Source: CAD feature listing. Evaluate the final solid. Frame: model axes, mm. Face numbers are marked on the shaded views. A direction names the side the tool comes from. Round coordinates to 2 decimals unless told otherwise and drop trailing zeros. Order: outer loops, then holes, each group sorted by start corner. A loop starts at its lowest first (then second) coordinate and runs counter-clockwise, first axis right, second up. Notation, with made-up numbers: M 30.5,89.25 L 59.5,89.25 A23 cw 59.5,126.25 Z; hole C 68,32.5 d9. An arc over 180 degrees is marked long. Answer as CSV lines item,"result". Start each with the question number.
Item 1: Section query B-B on z = 2.5. Return the cut outline in (x, y).
Item 2: Section query C-C on x = -8. Return the cut outline in (y, z), plus the area to 3 significant figures.
Item 3: Line query: line 1 (Y direction, x = 0, z = 37.5); line 2 (X direction, y = 4, z = 0); line 3 (X direction, y = 72, z = 22). Output: solid intervals per line, ascending. Write a range as [from, to].
Item 4: Section query A-A on x = -2.5. Return the cut outline in (y, z), plus the area to 3 significant figures.
Item 5: Section query D-D on y = 52.5. Return the cut outline in (x, z).
Item 6: Set-up query: the marked faces 1 and 2. Return all of +Z, -Z, +X, -X, +Y, -Y with unobstructed straight access to the full face (end or side cutting, diameter ignored); none if empty.
Item 7: First-contact query: P1, Ø10, axis at x = -1, y = 72.5, coming from the +Z side; P2, Ø8, axis at y = 36.5, z = -8.5, coming from the +X side; P3, Ø1, axis at x = -7.5, y = 29, coming from the +Z side. Flat tips, straight axial feed; report the tip coordinate or a pass-through.
Item 8: Pull-direction query (X, two-part tool) for the marked faces 3, 4 and 5; classes: +X half, -X half, draft (parallel to the pull), parting line (faces both ways), or undercut.
from build123d import *
from build123d.topology import SkipClean

# Parameters (mm, degrees)
SKETCH1_R           = 15.3
BOSS_EXTRUDE1_DEPTH = 84.864
SKETCH2_R           = 13.97
BOSS_EXTRUDE2_DEPTH = 57.15
BOSS_EXTRUDE3_DEPTH = 2.54
SKETCH4_R           = 10.2235
CUT_EXTRUDE1_DEPTH  = 5.08
SKETCH5_R           = 14.2621
SKETCH5_R_2         = 10.2235
BOSS_EXTRUDE4_DEPTH = 19.05
SKETCH6_R           = 10.75
CUT_EXTRUDE2_DEPTH  = 6.2
SKETCH8_R           = 14.2621
CUT_EXTRUDE5_DEPTH  = 10.16
SKETCH10_R          = 13.97
BOSS_EXTRUDE5_DEPTH = 24.13
SKETCH11_R          = 10.2235
CUT_EXTRUDE7_DEPTH  = 41.91
SKETCH13_R          = 14.2621
SKETCH13_R_2        = 10.2235
CUT_EXTRUDE9_DEPTH  = 41.91
SKETCH16_R          = 13.97
SKETCH16_R_2        = 10.2235
CUT_EXTRUDE10_DEPTH = 27.78125
SKETCH17_R          = 10.2235
CUT_EXTRUDE11_DEPTH = 27.686
SKETCH18_R          = 6.35
CUT_EXTRUDE12_DEPTH = 111.506


with BuildPart() as part:
    # Sketch1 → Boss-Extrude1 (new body)
    with BuildSketch(Plane(origin=(0, 0, 0), x_dir=(1, 0, 0), z_dir=(0, 1, 0))):
        with Locations(Location((0, 0, 0), (0, 0, 270))):
            Circle(SKETCH1_R)
    extrude(amount=BOSS_EXTRUDE1_DEPTH)

    # Sketch2 → Boss-Extrude2 (add)
    with BuildSketch(Plane.XY):
        with Locations(Location((0, 70.894, 0), (0, 0, 269.999999993))):
            Circle(SKETCH2_R)
    extrude(amount=BOSS_EXTRUDE2_DEPTH)

    # Sketch3 → Boss-Extrude3 (add, symmetric)
    with BuildSketch(Plane.XY.offset(57.15)):
        with BuildLine():
            Line((16.764, 70.894), (16.764, 40.838899717))
            ThreePointArc((16.764, 40.838899717), (0, 24.074899717), (-16.764, 40.838899717))
            Line((-16.764, 40.838899717), (-16.764, 70.894))
            ThreePointArc((-16.764, 70.894), (0, 87.658), (16.764, 70.894))
        make_face()
    extrude(amount=BOSS_EXTRUDE3_DEPTH, both=True)

    # Sketch4 → Cut-Extrude1 (cut)
    with BuildSketch(Plane.XY.offset(59.69)):
        with Locations((0, 40.838899717)):
            Circle(SKETCH4_R)
    extrude(amount=-CUT_EXTRUDE1_DEPTH, mode=Mode.SUBTRACT)

    # Sketch5 → Boss-Extrude4 (add, symmetric)
    with SkipClean():  # the faces are left unmerged after this step: merging them gives an invalid solid
        with BuildSketch(Plane(origin=(0, 0, 54.61), x_dir=(-1, 0, 0), z_dir=(0, 0, -1))):
            with Locations(Location((0, 40.838899717, 0), (0, 0, 180))):
                Circle(SKETCH5_R)
            with Locations((0, 40.838899717)):
                Circle(SKETCH5_R_2, mode=Mode.SUBTRACT)
        extrude(amount=BOSS_EXTRUDE4_DEPTH, both=True)

    # Sketch6 → Cut-Extrude2 (cut)
    with SkipClean():  # the faces are left unmerged after this step: merging them gives an invalid solid
        with BuildSketch(Plane.XZ):
            with Locations(Location((0, 0, 0), (0, 0, 270))):
                Circle(SKETCH6_R)
        extrude(amount=-CUT_EXTRUDE2_DEPTH, mode=Mode.SUBTRACT)

    # Sketch8 → Cut-Extrude5 (cut)
    with SkipClean():  # the faces are left unmerged after this step: merging them gives an invalid solid
        with BuildSketch(Plane.XY.offset(59.69)):
            with BuildLine():
                Line((-16.764, 70.894), (-16.764, 40.838899717))
                ThreePointArc((-16.764, 40.838899717), (0, 24.074899717), (16.764, 40.838899717))
                Line((16.764, 40.838899717), (16.764, 70.894))
                ThreePointArc((16.764, 70.894), (0, 87.658), (-16.764, 70.894))
            make_face()
            with Locations((0, 40.838899717)):
                Circle(SKETCH8_R, mode=Mode.SUBTRACT)
        extrude(amount=-CUT_EXTRUDE5_DEPTH, mode=Mode.SUBTRACT)


with BuildPart() as cut_extrude5_piece_1:
    # of the separate pieces the step leaves, piece 1, a body of its own (cut_extrude5_pieces)
    add(part.part.solids().sort_by_distance((0, 0, 15.3))[0])

    # Sketch10 → Boss-Extrude5 (add)
    with BuildSketch(Plane.XY.offset(49.53)):
        with Locations(Location((0, 70.894, 0), (0, 0, 90))):
            Circle(SKETCH10_R)
    extrude(amount=BOSS_EXTRUDE5_DEPTH)

    # Sketch11 → Cut-Extrude7 (cut)
    with BuildSketch(Plane.XY.offset(73.66)):
        with Locations((0, 70.894)):
            Circle(SKETCH11_R)
    extrude(amount=-CUT_EXTRUDE7_DEPTH, mode=Mode.SUBTRACT)

    # Sketch16 → Cut-Extrude10 (cut)
    with BuildSketch(Plane.XY.offset(73.66)):
        with Locations(Location((0, 70.894, 0), (0, 0, 90))):
            Circle(SKETCH16_R)
        with Locations((0, 70.894)):
            Circle(SKETCH16_R_2, mode=Mode.SUBTRACT)
    extrude(amount=-CUT_EXTRUDE10_DEPTH, mode=Mode.SUBTRACT)

    # Sketch17 → Cut-Extrude11 (cut)
    with BuildSketch(Plane.XY.offset(31.75)):
        with Locations((0, 70.894)):
            Circle(SKETCH17_R)
    extrude(amount=-CUT_EXTRUDE11_DEPTH, mode=Mode.SUBTRACT)

    # Sketch18 → Cut-Extrude12 (cut)
    with BuildSketch(Plane.XY.offset(4.064)):
        with Locations((0, 70.894)):
            Circle(SKETCH18_R)
    extrude(amount=-CUT_EXTRUDE12_DEPTH, mode=Mode.SUBTRACT)


with BuildPart() as cut_extrude5_piece_2:
    # of the separate pieces the step leaves, piece 2, a body of its own (cut_extrude5_pieces)
    add(part.part.solids().sort_by_distance((14.2621, 40.838899717, 54.61))[0])

    # Sketch13 → Cut-Extrude9 (cut)
    with BuildSketch(Plane.XY.offset(73.66)):
        with Locations((0, 40.838899717)):
            Circle(SKETCH13_R)
        with Locations((0, 40.838899717)):
            Circle(SKETCH13_R_2, mode=Mode.SUBTRACT)
    extrude(amount=-CUT_EXTRUDE9_DEPTH, mode=Mode.SUBTRACT)


solid = cut_extrude5_piece_1.part
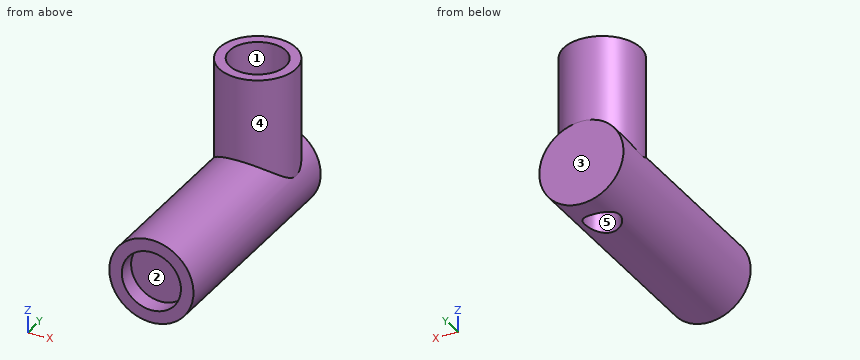
Results:
1,outline,"M -15.09,0 L -10.46,0 L -10.46,6.2 L 10.46,6.2 L 10.46,0 L 15.09,0 L 15.09,84.86 L -15.09,84.86 Z; hole C 0,70.89 d12.7"
2,outline,"M 0,-13.04 L 84.86,-13.04 L 84.86,13.04 L 82.35,13.04 L 82.35,45.88 L 77.26,45.88 L 77.26,4.06 L 64.53,4.06 L 64.53,45.88 L 59.44,45.88 L 59.44,13.04 L 0,13.04 L 0,7.18 L 6.2,7.18 L 6.2,-7.18 L 0,-7.18 Z"
2,area,"2,340 mm^2"
3,line 1,"[56.92, 60.67], [81.12, 84.86]"
3,line 2,"[-15.3, -10.75], [10.75, 15.3]"
3,line 3,"[-13.93, -10.16], [10.16, 13.93]"
4,outline,"M 0,-15.09 L 65.06,-15.09 L 65.06,4.06 L 60.98,4.06 L 60.98,45.88 L 57.15,45.88 L 57.15,15.09 L 0,15.09 L 0,10.46 L 6.2,10.46 L 6.2,-10.46 L 0,-10.46 Z; M 76.73,-15.09 L 84.86,-15.09 L 84.86,15.09 L 84.64,15.09 L 84.64,45.88 L 80.81,45.88 L 80.81,4.06 L 76.73,4.06 Z"
4,area,"2,230 mm^2"
5,outline,"C 0,0 d30.6"
6,face 1,"+Z"
6,face 2,"-Y"
7,P1,"z = 4.06"
7,P2,"x = 14.62"
7,P3,"z = 13.6"
8,face 3,"draft"
8,face 4,"parting line"
8,face 5,"undercut"
